Geometry: see drawing. Coordinates: mm, zero at the bounding-box minimum. A direction names the side the tool comes from. Coordinates: 2 decimals unless noted, no trailing zeros. Order: outer loops, then holes, each group sorted by start corner. A loop starts at its lowest first (then second) coordinate and runs counter-clockwise, first axis right, second up. Notation, with made-up numbers: (-29, 22.25) -> (29, 22.25) arc R24 cw to (29, 57.25) -> close; hole circle Ø5 at (-14, 78.5). An arc over 180 degrees is marked (long way). Write each question's results on one line, items separated by ' | '. Start each with the question number.
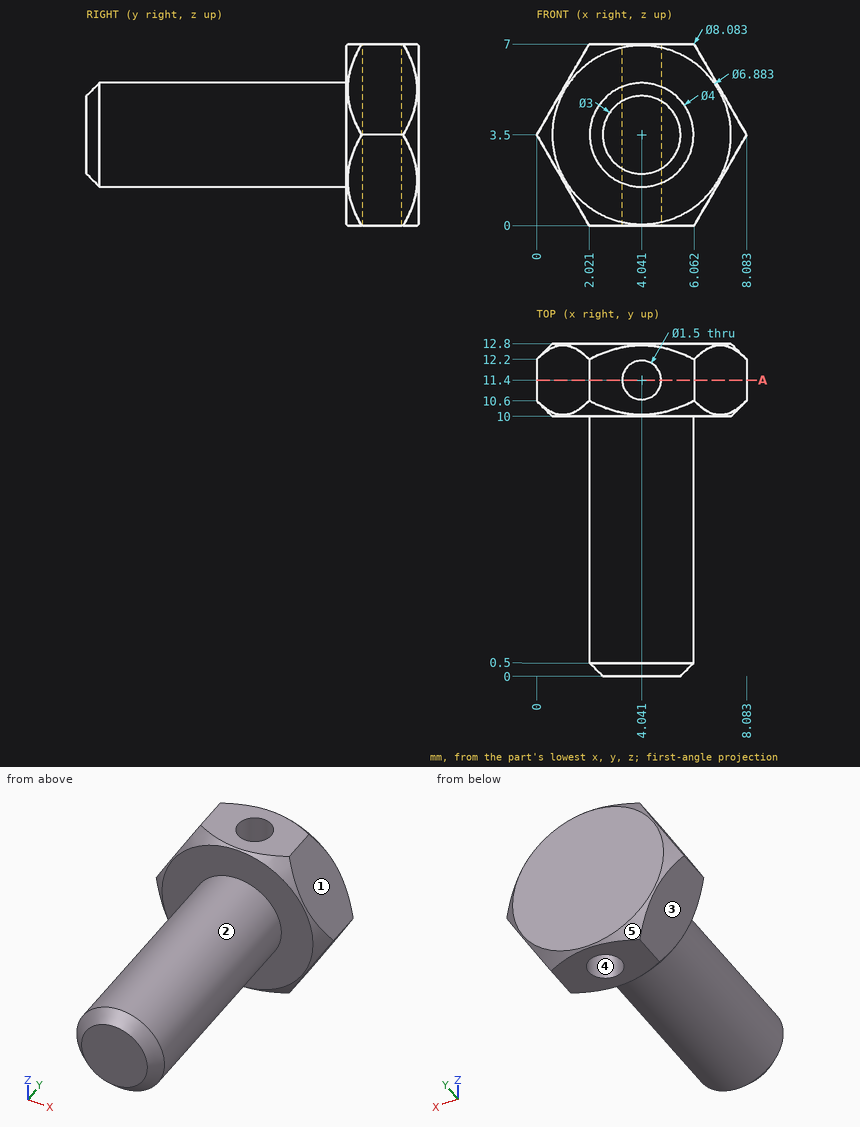
(1) Section A-A on y = 11.4. Return the cut outline in (x, z).
(2) Reachability of the marked faces 1 and 2 from +Z, -Z, +X, -X, +Y, -Y: full face, straight path, thin tool, end or side. Return the list, or none.
(3) Line query: L1, parallel to Y at x = 6.75, z = 5; L2, parallel to X at y = 10.75, z = 2.25 (1 decimal); L3, parallel to Y at x = 3.75, z = 1. Output: solid intervals per line, ascending.
(4) Draft query along X for the marked faces 3, 4 and 5. Return one class per face: released by +X, released by -X, zero draft, split by the parting line, or undercut.
(5) First-contact query: P1, Ø1, axis at x = 5.5, z = 3, coming from the -Y side; P2, Ø3, axis at y = 6, z = 1.5, coming from the +X side. Flat tips, straight axial feed; report the tip coordinate or a pass-through.
Results list:
1) outline: (0, 3.5) -> (2.02, 0) -> (3.29, 0) -> (3.29, 7) -> (2.02, 7) -> close; (4.79, 0) -> (6.06, 0) -> (8.08, 3.5) -> (6.06, 7) -> (4.79, 7) -> close
2) face 1: +Z, +X, +Y, -Y | face 2: -Y
3) L1: y = 10 to 12.8 | L2: x = 0.7 to 3.7, 4.4 to 7.4 | L3: y = 10 to 10.71, 12.09 to 12.8
4) face 3: released by -X | face 4: undercut | face 5: split by the parting line
5) P1: stops at y = 0 | P2: stops at x = 5.98
